The model under review builds one solid part; all positions refer to its coordinate system, in mm. A direction names the side the tool comes from. Coordinates: 2 decimals unless noted, no trailing zeros. Loops run counter-clockwise (first coordinate to the right, second up) from the corner with the lowest first, then second, coordinate; pieces in that order, holes last. Notation, with made-up numbers: (23, 79.25) - (56, 79.25) arc R20 cw to (56, 115.25) - close; hole circle Ø3 at (34, -24.75). An arc over 180 degrees is marked (long way). Answer in a Markdown table with one row per item. Add a question column.
(1) For P1, Ø15.5, axis at x = -87, y = -69, coming from the +Z side; P2, Ø2, axis at x = -97.5, z = 42.5, coming from the +Y side; P3, Ø12, axis at x = -23.5, y = -64, coming from the -Z side; P4, Ø5, axis at x = -40.5, y = -32.5, coming from the +Z side, all flat-tipped, find the tip position at first contact; note any pin that passes through.
(2) We need section C-C on y = -60.5. Write out the cut boundary in (x, z).
(3) Mouldability with a two-part tool opening along Z and no side actions: class faces 1 (the flat face through (-50, -38, 0)), 2 (the cylindrical face through (-55.281, -63.616, 36.926)), 3 (the flat face through (-84, -50, 76.2)), 4 (the flat face through (-97, 0, 38)) as +Z half, -Z half, draft (parallel to the pull), parting line (faces both ways), or undercut.
(4) For line 1 along Y through (x, z) = (-62.5, 74); line 2 along Z through (x, y) = (-79, -53.5); line 3 along Z through (x, y) = (-42, -12), list the stretches that pass through material, from the lowest coordinate up.
(5) Machinability: for faces 5 (the flat face through (-47.35, -40.22, 47.38)), 6 (the flat face through (-59, 24.076, 34)), 7 (the flat face through (-94.828, 12, 44)), 8 (the flat face through (-59.88, -52.52, 21.18)), 9 (the flat face through (-31.73, 11.87, 45.18)), which of the approach directions +Z, -Z, +X, -X, +Y, -Y give a long, thin tool a straight path to every point of the face, cutting with its end or side? Answer none if there is none.
(6) We need section A-A on x = -90. Write out the cut boundary in (y, z).
(7) We need section B-B on y = -3.5. Write out the cut boundary in (x, z), plus the area to 3 significant figures.
(8) We need section D-D on x = -12. Write out the cut boundary in (y, z), plus the area to 3 significant figures.
from build123d import *

# Parameters (mm, degrees)
F0_W     = 94.8279574513
F0_H     = 24.0764599293
F1_DEPTH = 88.9
F3_DEPTH = 49.022
F4_W     = 84.5879163432
F4_H     = 101.6
F5_DEPTH = 76.2
F7_DEPTH = 101.6
F8_R     = 15.3482733218
F9_DEPTH = 25.4


with BuildPart() as f1:
    # F0 (on Top) → F1 (new body)
    with BuildSketch(Plane.XY):
        with Locations((-47.4139787257, 12.0382299647)):
            Rectangle(F0_W, F0_H)
    extrude(amount=F1_DEPTH)

    # F2 (on face) → F3 (cut)
    with BuildSketch(Plane.XZ):
        Polygon((0, 88.9), (-62.5919832129, 88.9), (0, 0.2280238973), align=None)
    extrude(amount=-F3_DEPTH, mode=Mode.SUBTRACT)

    # F4 (on Top) → F5 (join)
    with BuildSketch(Plane.XY):
        with Locations((-56.447530406, -50.8)):
            Rectangle(F4_W, F4_H)
    extrude(amount=F5_DEPTH)

    # F6 (on face) → F7 (cut)
    with BuildSketch(Plane.XZ.offset(101.6)):
        Polygon((-14.1535722344, 76.2), (-67.8575116148, 76.2), (-14.1535722344, 0.7241950249), align=None)
    extrude(amount=-F7_DEPTH, mode=Mode.SUBTRACT)

    # F8 (on face) → F9 (cut)
    with BuildSketch(Plane(origin=(-9.054237048, 0, -6.4424380465), x_dir=(0, 1, 0), z_dir=(0.814790835, 0, 0.5797550304))):
        with Locations((-52.3036755621, 51.7632775009)):
            Circle(F8_R)
    extrude(amount=-F9_DEPTH, mode=Mode.SUBTRACT)


solid = f1.part
Outcome:
| question | item | result |
|---|---|---|
| 1 | P1 | z = 76.2 |
| 1 | P2 | y = 0 |
| 1 | P3 | z = 0 |
| 1 | P4 | z = 41.27 |
| 2 | outline | (-98.74, 0) - (-14.15, 0) - (-14.15, 0.72) - (-31.54, 25.16) - (-52.24, 10.43) - (-67.28, 31.58) - (-46.59, 46.31) - (-67.86, 76.2) - (-98.74, 76.2) - close |
| 3 | face 1 | -Z half |
| 3 | face 2 | undercut |
| 3 | face 3 | +Z half |
| 3 | face 4 | draft |
| 4 | line 1 | 0 to 24.08 |
| 4 | line 2 | 0 to 76.2 |
| 4 | line 3 | 0 to 39.86 |
| 5 | face 5 | +Z, +X, -Y |
| 5 | face 6 | +Z, -Z, +X, -X, +Y |
| 5 | face 7 | +Z, -Z, -X, +Y |
| 5 | face 8 | none |
| 5 | face 9 | +Z, +X, +Y, -Y |
| 6 | outline | (-101.6, 0) - (24.08, 0) - (24.08, 88.9) - (0, 88.9) - (0, 76.2) - (-101.6, 76.2) - close |
| 7 | outline | (-98.74, 0) - (-14.15, 0) - (-14.15, 0.72) - (-67.86, 76.2) - (-98.74, 76.2) - close |
| 7 | area | 4,420 mm² |
| 8 | outline | (0, 0) - (24.08, 0) - (24.08, 17.23) - (0, 17.23) - close |
| 8 | area | 415 mm² |
